Build history of the part. All positions in model axes, mm. Give positions to 0.01 mm unless a question says otherwise; leave off trailing zeros. Loops run counter-clockwise (first coordinate to the right, second up) from the corner with the lowest first, then second, coordinate; pieces in that order, holes last. Notation, with made-up numbers: (51.5, 18.25) -> (105.5, 18.25) arc R23 ccw to (105.5, 55.25) -> close; hole circle Ø1 at (66.5, 55). An arc over 180 degrees is marked (long way). Answer as a JSON object with one key per item and string values. Group by question number.
Q1. Band-saw the part on B-B, the plane x = -91. Write the cut outline in (y, z).
Q2. Wall check: probe 1 along Z at (x, y) = (-80.5, 2.5); probe 2 along X at (y, z) = (-1.75, 25.5); probe 3 along Z at (x, y) = (-75, 3). Give the ranges that are in metal, low to high. Write a range as from..to.
Q3. Band-saw the part on A-A, the plane y = -3. Count the separate pieces of the cut face and the enclosed holes in it, plus the area to 3 significant figures.
Q4. Band-saw the part on D-D, the plane z = 8. Write the cut outline in (x, y).
Q5. Drop flat-ended pins along their axis: pin 1 (3.5 mm diameter, centred on x = -80.76, z = 53.73, fed in from +Y); pin 2 (1.8 mm diameter, centred on x = -95.17, z = 18.74, fed in from +Y); pin 3 (3 mm diameter, centred on y = 1.5, z = 47, fed in from -X); pin 4 (2 mm diameter, centred on y = 0.5, z = 11.5, fed in from -X). Give the stop position or say it passes through.
Q6. Band-saw the part on C-C, the plane z = 16. Write the cut outline in (x, y).
Q7. Two-plate mould, pull along Z, no slides. Class faces 1 (the flat face through (-88, 1.5, 38)), 2 (the cylindrical face through (-87.041, -2.732, 35.494)), 3 (the flat face through (-71, 0, 71)), 4 (the cylindrical face through (-95.28, 2.77, 20.23)): pulls with the +Z half, pulls with the -Z half, needs draft (parallel to the pull), parting line crosses it, or undercut.
from build123d import *

# Parameters (mm, degrees)
R_VOLUTION1_ANGLE            = 45
ESQUISSE3_R                  = 1.5
ENL_V_MAT_EXTRU_1_DEPTH      = 9
R_P_TITION_CIRCULAIRE1_COUNT = 10
R_P_TITION_CIRCULAIRE1_ANGLE = 40.5


with BuildPart() as part:
    # Esquisse2 → Révolution1 (revolve)
    with BuildSketch(Plane.XY):
        Polygon((-103, 4), (-103, -4), (-94, -4), (-94, -1.5), (-100, -1.5), (-100, 1.5), (-94, 1.5), (-94, 4), align=None)
    revolve(axis=Axis((0, -55, 0), (0, 1, 0)), revolution_arc=R_VOLUTION1_ANGLE)

    # Esquisse3 → Enlèv. mat.-Extru.1 (cut, through all)
    with BuildSketch(Plane(origin=(0, 4, 0), x_dir=(1, 0, 0), z_dir=(0, 1, 0))):
        with Locations((-71.359442001, -65.702587752)):
            Circle(ESQUISSE3_R)
    enl_v_mat_extru_1 = extrude(amount=-ENL_V_MAT_EXTRU_1_DEPTH, mode=Mode.SUBTRACT)

    # Répétition circulaire1: Enlèv. mat.-Extru.1 ×10 about axis
    r_p_tition_circulaire1_axis = Axis((0, 0, 0), (0, -1, 0))
    for i in range(1, R_P_TITION_CIRCULAIRE1_COUNT):
        add(enl_v_mat_extru_1.rotate(r_p_tition_circulaire1_axis, i * R_P_TITION_CIRCULAIRE1_ANGLE / (R_P_TITION_CIRCULAIRE1_COUNT - 1)), mode=Mode.SUBTRACT)


solid = part.part
Worked answers:
{
 "1": {"outline": "(-4, 23.56) -> (-1.5, 23.56) -> (-1.5, 31.89) -> (-4, 31.89) -> close; (-4, 34.89) -> (-1.5, 34.89) -> (-1.5, 41.46) -> (1.5, 41.46) -> (1.5, 34.89) -> (4, 34.89) -> (4, 48.25) -> (-4, 48.25) -> close; (1.5, 23.56) -> (4, 23.56) -> (4, 31.89) -> (1.5, 31.89) -> close"},
 "2": {"probe 1": "48.54..52.25, 55.21..64.26", "probe 2": "-99.79..-94.76, -92.06..-90.48", "probe 3": "56.67..59.14, 60.66..70.6"},
 "3": {"separate pieces": "1", "enclosed holes": "10", "area": "626 mm2"},
 "4": {"outline": "(-102.69, -4) -> (-93.66, -4) -> (-93.66, -1.5) -> (-99.68, -1.5) -> (-99.68, 1.5) -> (-93.66, 1.5) -> (-93.66, 4) -> (-102.69, 4) -> close"},
 "5": {"pin 1": "y = 4", "pin 2": "through", "pin 3": "x = -92.41", "pin 4": "x = -102.46"},
 "6": {"outline": "(-101.75, -4) -> (-92.63, -4) -> (-92.63, -1.5) -> (-98.71, -1.5) -> (-98.71, 1.5) -> (-92.63, 1.5) -> (-92.63, 4) -> (-101.75, 4) -> close"},
 "7": {"face 1": "needs draft", "face 2": "pulls with the -Z half", "face 3": "pulls with the +Z half", "face 4": "undercut"}
}
